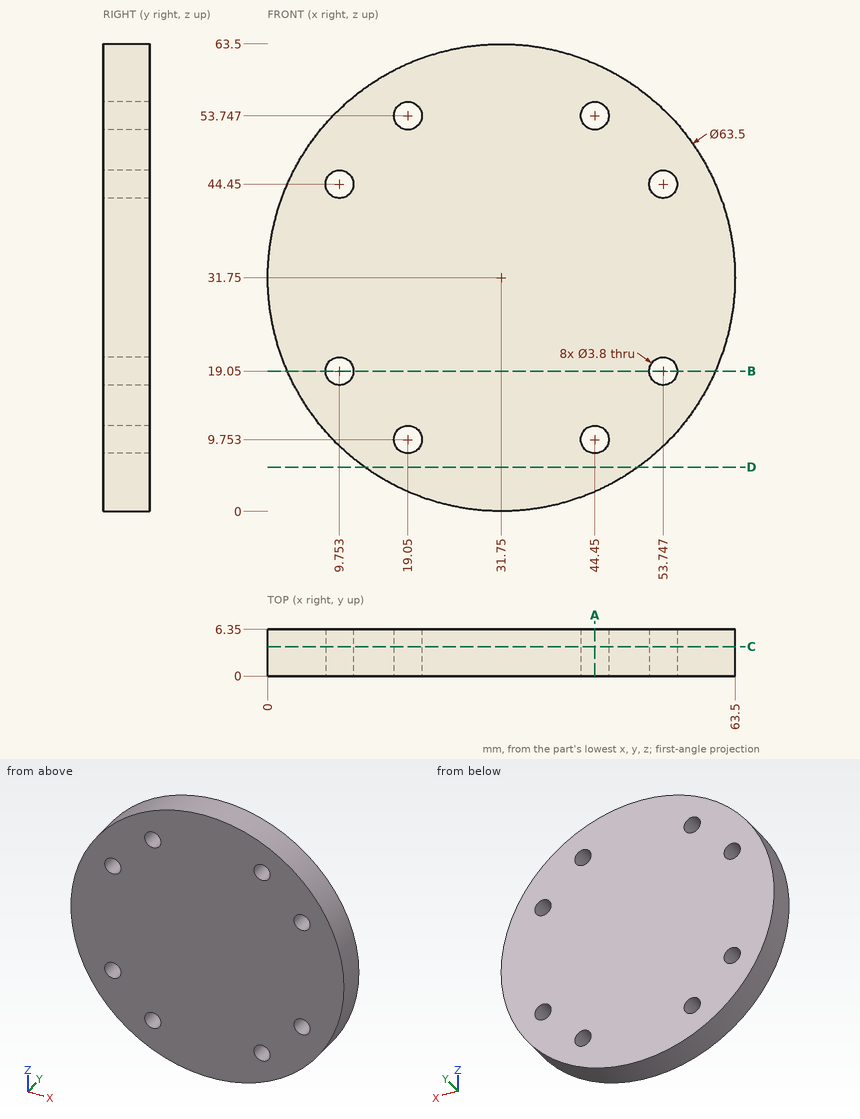
The drawing under review shows one solid part. Ordinate dimensions are in mm from its lowest x, y, z. Coordinates: 2 decimals unless noted, no trailing zeros. Write each loop counter-clockwise with the first axis right and the second up, starting at its lowest first coordinate (ties: lowest second). Pieces come first, ordered by that corner, then holes. Notation, with made-up numbers: (-27.75, -27.75) - (4.25, -27.75) arc R12 ccw to (4.25, -7.75) - close; hole circle Ø10 at (64, -7). An arc over 180 degrees is marked (long way). Put each result on its own line as item: value.
1. For pin 1 (1.5 mm diameter, centred on y = 2.5, z = 12, fed in from -X); pin 2 (1 mm diameter, centred on x = 12.5, y = 3, fed in from +Z); pin 3 (2 mm diameter, centred on y = 5.5, z = 22.5, fed in from +X), all flat-tipped, find the tip position at first contact; note any pin that passes through.
Values found:
pin 1: x = 6.31
pin 2: z = 57.37
pin 3: x = 62.41
2. Add section C-C, the plane y = 4. Count the separate pieces of the cut face and the enclosed holes in it, then the cut area to 3 significant figures.
Values found:
separate pieces: 1
enclosed holes: 8
area: 3,080 mm²
3. Wall thickness on probe 1 along Z at (x, y) = (44.45, 3.25); probe 2 along Z at (x, y) = (17.5, 2); probe 3 along X at (y, z) = (3.25, 54): over which ranges is each line inside the solid? List them lowest first.
Values found:
probe 1: 2.65 to 7.85, 11.65 to 51.85, 55.65 to 60.85
probe 2: 3.38 to 8.65, 10.85 to 52.65, 54.85 to 60.12
probe 3: 9.1 to 17.17, 20.93 to 42.57, 46.33 to 54.4
4. Add section D-D, the plane z = 6. Give the boundary of the cut face in (x, y), then the cut area to 3 significant figures.
Values found:
outline: (13.18, 0) - (50.32, 0) - (50.32, 6.35) - (13.18, 6.35) - close
area: 236 mm²
5. Add section A-A, the plane x = 44.45. Give the boundary of the cut face in (y, z), then the cut area to 3 significant figures.
Values found:
outline: (0, 2.65) - (6.35, 2.65) - (6.35, 7.85) - (0, 7.85) - close; (0, 11.65) - (6.35, 11.65) - (6.35, 51.85) - (0, 51.85) - close; (0, 55.65) - (6.35, 55.65) - (6.35, 60.85) - (0, 60.85) - close
area: 321 mm²
6. Add section B-B, the plane z = 19.05. Give the boundary of the cut face in (x, y), then the cut area to 3 significant figures.
Values found:
outline: (2.65, 0) - (7.85, 0) - (7.85, 6.35) - (2.65, 6.35) - close; (11.65, 0) - (51.85, 0) - (51.85, 6.35) - (11.65, 6.35) - close; (55.65, 0) - (60.85, 0) - (60.85, 6.35) - (55.65, 6.35) - close
area: 321 mm²
